from build123d import *

# Parameters (mm, degrees)
F1_DEPTH = 25.4
F2_DEPTH = 12.7
F3_R     = 9.3751640111
F4_DEPTH = 12.7
F5_DEPTH = 38.101


with BuildPart() as f1:
    # F0 (on Top) → F1 (new body)
    with BuildSketch(Plane.XY):
        with BuildLine():
            Line((32.6498188078, -5.9798206203), (19.062470553, 48.6717349119))
            ThreePointArc((19.062470553, 48.6717349119), (-1.2334703342, 52.2374412428), (-21.2233329751, 47.2329562812))
            Line((-21.2233329751, 47.2329562812), (-27.0181472742, -5.9798206203))
            Line((-27.0181472742, -5.9798206203), (-11.8400434842, -5.9798206203))
            Line((-11.8400434842, -5.9798206203), (-4.9034534022, 13.8731840998))
            Line((-4.9034534022, 13.8731840998), (9.4984725438, 13.8731840998))
            Line((9.4984725438, 13.8731840998), (15.767841556, -5.9798206203))
            Line((15.767841556, -5.9798206203), (32.6498188078, -5.9798206203))
        make_face()
    extrude(amount=F1_DEPTH)

    # F0 (on Top) + F1_face (on face) → F2 (join, symmetric)
    with BuildSketch(Plane.XY):
        with BuildLine():
            Line((32.6498188078, -5.9798206203), (19.062470553, 48.6717349119))
            ThreePointArc((19.062470553, 48.6717349119), (-1.2334703342, 52.2374412428), (-21.2233329751, 47.2329562812))
            Line((-21.2233329751, 47.2329562812), (-27.0181472742, -5.9798206203))
            Line((-27.0181472742, -5.9798206203), (-11.8400434842, -5.9798206203))
            Line((-11.8400434842, -5.9798206203), (-4.9034534022, 13.8731840998))
            Line((-4.9034534022, 13.8731840998), (9.4984725438, 13.8731840998))
            Line((9.4984725438, 13.8731840998), (15.767841556, -5.9798206203))
            Line((15.767841556, -5.9798206203), (32.6498188078, -5.9798206203))
        make_face()
    with BuildSketch(Plane(origin=(0.8435409234, 23.5753340068, 25.4), x_dir=(1, 0, 0), z_dir=(0, 0, 1))):
        with BuildLine():
            Line((31.8062778844, -29.5551546271), (18.2189296295, 25.0964009052))
            ThreePointArc((18.2189296295, 25.0964009052), (-2.0770112576, 28.662107236), (-22.0668738986, 23.6576222744))
            Line((-22.0668738986, 23.6576222744), (-27.8616881976, -29.5551546271))
            Line((-27.8616881976, -29.5551546271), (-12.6835844076, -29.5551546271))
            Line((-12.6835844076, -29.5551546271), (-5.7469943256, -9.702149907))
            Line((-5.7469943256, -9.702149907), (8.6549316203, -9.702149907))
            Line((8.6549316203, -9.702149907), (14.9243006326, -29.5551546271))
            Line((14.9243006326, -29.5551546271), (31.8062778844, -29.5551546271))
        make_face()
    extrude(amount=F2_DEPTH, both=True)

    # F3 (on face) → F4 (cut, symmetric)
    with BuildSketch(Plane.XY.offset(38.1)):
        with Locations((0, 32.7694192529)):
            Circle(F3_R)
    extrude(amount=F4_DEPTH, both=True, mode=Mode.SUBTRACT)

    # F5 (cut, through all): a face of the model
    f5_faces = [f1.faces().sort_by_distance(p)[0] for p in [
        (0, 32.7694192529, 25.4),
    ]]
    extrude(f5_faces, amount=-F5_DEPTH, mode=Mode.SUBTRACT)


solid = f1.part
Input: part model. Units: mm. Frame: model coordinates. A direction names the side the tool comes from. Give positions to 0.01 mm unless a question says otherwise; leave off trailing zeros. Write each loop counter-clockwise with the first axis right and the second up, starting at its lowest first coordinate (ties: lowest second). Pieces come first, ordered by that corner, then holes.
Q1. Section A-A, the plane y = 4. Output: boundary loops of the cut face in (x, z).
Q2. Pull-direction query (X, two-part tool) for faces 1 (the face through (-0.943, 52.247, 12.344)), 2 (the face through (-8.42, 3.81, 12.34)), 3 (the face through (2.4, 23.55, 38.1)); classes: pulls with the +X half, pulls with the -X half, needs draft (parallel to the pull), parting line crosses it, or undercut.
Q3. First-contact query: P1, Ø4.5, axis at x = 4.5, z = 5.5, coming from the -Y side; P2, Ø1.5, axis at y = 19.5, z = 16, coming from the -X side; P3, Ø10, axis at x = 5, y = 31, coming from the +Z side; P4, Ø10, axis at x = 6, z = -2, coming from the +Y side. Flat tips, straight axial feed; report the tip coordinate or a pass-through.
Q4. Set-up query: faces 4 (the face through (2.4, 23.55, -12.7)), 5 (the face through (2, 13.873, 13)). Return all of +Z, -Z, +X, -X, +Y, -Y with unobstructed straight access to the full face (end or side cutting, diameter ignored); none if empty.
Q5. Section C-C, the plane z = 35. Output: boundary loops of the cut face in (x, y), plus the area to 3 significant figures.
Q6. Section D-D, the plane x = 23.5. Output: boundary loops of the cut face in (y, z).
Q7. Section B-B, the plane x = 0. Output: boundary loops of the cut face in (y, z), plus the area to 3 significant figures.
Q8. Material intervals for probe 1 along Y at (x, z) = (0, 10); probe 2 along X at (y, z) = (-1, 36); probe 3 along X at (y, z) = (32.5, 25), sorted ascending.
Filled in:
1. outline: (-25.93, -12.7) - (-8.35, -12.7) - (-8.35, 38.1) - (-25.93, 38.1) - close; (12.62, -12.7) - (30.17, -12.7) - (30.17, 38.1) - (12.62, 38.1) - close
2. face 1: parting line crosses it
2. face 2: undercut
2. face 3: needs draft
3. P1: stops at y = 13.87
3. P2: stops at x = -24.33
3. P3: stops at z = 38.1
3. P4: stops at y = 52.27
4. face 4: -Z, +X, -X, +Y, -Y
4. face 5: +Z, -Z, -Y
5. outline: (-27.02, -5.98) - (-11.84, -5.98) - (-4.9, 13.87) - (9.5, 13.87) - (15.77, -5.98) - (32.65, -5.98) - (19.06, 48.67) arc R49.52 ccw to (-21.22, 47.23) - close; hole circle Ø18.75 at (0, 32.77)
5. area: 2,120 mm2
6. outline: (-5.98, -12.7) - (30.82, -12.7) - (30.82, 38.1) - (-5.98, 38.1) - close
7. outline: (13.87, -12.7) - (23.39, -12.7) - (23.39, 38.1) - (13.87, 38.1) - close; (42.14, -12.7) - (52.27, -12.7) - (52.27, 38.1) - (42.14, 38.1) - close
7. area: 998 mm2
8. probe 1: y = 13.87 to 23.39, 42.14 to 52.27
8. probe 2: x = -26.48 to -10.1, 14.2 to 31.41
8. probe 3: x = -22.83 to -9.37, 9.37 to 23.08
